```python
from build123d import *

# Parameters (mm, degrees)
SKETCH1_R           = 15.875
BOSS_EXTRUDE1_DEPTH = 19.05


with BuildPart() as part:
    # Sketch1 → Boss-Extrude1 (new body)
    with BuildSketch(Plane.XY):
        with BuildLine():
            Line((33.072437746, -6.234812473), (12.7, -114.3))
            Line((12.7, -114.3), (-88.9, -114.3))
            Line((-88.9, -114.3), (-30.640469546, 13.921948535))
            ThreePointArc((-30.640469546, 13.921948535), (10.151471367, 32.087484384), (33.072437746, -6.234812473))
        make_face()
        Circle(SKETCH1_R, mode=Mode.SUBTRACT)
    extrude(amount=BOSS_EXTRUDE1_DEPTH)


solid = part.part
```
Geometry: final body of the model. Coordinates: model frame, mm. Round coordinates to 2 decimals unless told otherwise and drop trailing zeros. Order: outer loops, then holes, each group sorted by start corner. A loop starts at its lowest first (then second) coordinate and runs counter-clockwise, first axis right, second up. Notation, with made-up numbers: (79, 71) - (118, 71) arc R21 cw to (118, 105) - close; hole circle Ø3 at (4, 38.5). An arc over 180 degrees is marked (long way). Use CSV: the item, a comma, the result in double quotes. Start each with the question number.
Q1. Section query A-A (x = 0). Return loops of the section in (y, z) (3 decimals), and give its area (3 significant figures).
Q2. Section query B-B (z = 15.75). Return loops of the section in (x, y) (3 decimals).
Q3. Mould query, pull axis X, two halves, no side actions, for faces 1 (the face through (9.498, 32.287, 9.392)), 2 (the face through (-60.18, -51.09, 9.39)), 3 (the face through (23.03, -59.51, 9.39)), 4 (the face through (-3.441, -15.497, 9.392)). Classes: +X half, -X half, draft (parallel to the pull), parting line (faces both ways), or undercut.
Q4. Section query C-C (y = -4.5). Return loops of the section in (x, z).
Q5. Material intervals for line 1 along Y through (x, z) = (0, 4.25) (3 decimals); line 2 along Y through (x, z) = (-8.5, 7); line 3 along X through (y, z) = (19, 5.75), sorted ascending. Write a range as from..to.
Q6. Section query D-D (x = 18.5). Return loops of the section in (y, z), and give its area (3 significant figures).
Q7. First-contact query: pin 1 (1.5 mm diameter, centred on y = 5.5, z = 8, fed in from -X); pin 2 (4 mm diameter, centred on x = -55, z = 10.5, fed in from +Y); pin 3 (4 mm diameter, centred on y = -14.5, z = 2.5, fed in from +X). Flat tips, straight axial feed; report the tip coordinate or a pass-through.
Result set:
1,outline,"(-114.3, 0) - (-15.875, 0) - (-15.875, 19.05) - (-114.3, 19.05) - close; (15.875, 0) - (33.655, 0) - (33.655, 19.05) - (15.875, 19.05) - close"
1,area,"2,210 mm2"
2,outline,"(-88.9, -114.3) - (12.7, -114.3) - (33.072, -6.235) arc R33.655 ccw to (-30.64, 13.922) - close; hole circle Ø31.75 at (0, 0)"
3,face 1,"parting line"
3,face 2,"-X half"
3,face 3,"+X half"
3,face 4,"undercut"
4,outline,"(-39.01, 0) - (-15.22, 0) - (-15.22, 19.05) - (-39.01, 19.05) - close; (15.22, 0) - (33.35, 0) - (33.35, 19.05) - (15.22, 19.05) - close"
5,line 1,"y = -114.3..-15.875, 15.875..33.655"
5,line 2,"y = -114.3..-13.41, 13.41..32.56"
5,line 3,"x = -27.78..27.78"
6,outline,"(-83.53, 0) - (28.11, 0) - (28.11, 19.05) - (-83.53, 19.05) - close"
6,area,"2,130 mm2"
7,pin 1,"stops at x = -34.81"
7,pin 2,"stops at y = -35.29"
7,pin 3,"stops at x = 31.89"
